CAD build for the part. Positions are in the model's coordinates, mm. Face numbers are marked on the shaded views. A direction names the side the tool comes from. Give positions to 0.01 mm unless a question says otherwise; leave off trailing zeros. Write each loop counter-clockwise with the first axis right and the second up, starting at its lowest first coordinate (ties: lowest second). Pieces come first, ordered by that corner, then holes. Notation, with made-up numbers: (-14.75, 30.25) -> (44.25, 30.25) arc R20 ccw to (44.25, 58.25) -> close; hole circle Ø5 at (72, -23). An arc over 180 degrees is marked (long way). Answer as a JSON object with one key per item and string values.
```python
from build123d import *

# Parameters (mm, degrees)
BOSS_EXTRUDE1_DEPTH                      = 38
BOSS_EXTRUDE3_DEPTH                      = 26
FILLET1_R                                = 6
CBORE_FOR_M30_HEX_HEAD_BOLT2_D           = 38
CBORE_FOR_M30_HEX_HEAD_BOLT2_CBORE_D     = 57
CBORE_FOR_M30_HEX_HEAD_BOLT2_CBORE_DEPTH = 1
SKETCH17_W                               = 26
SKETCH17_H                               = 18.384776311
CUT_EXTRUDE3_DEPTH                       = 180.605122421


with BuildPart() as part:
    # Sketch1 → Boss-Extrude1 (new body, symmetric)
    with BuildSketch(Plane.XY):
        Polygon((38, 139), (127, 50), (127, 0), (0, 0), (0, 139), align=None)
    extrude(amount=BOSS_EXTRUDE1_DEPTH, both=True)

    # Sketch3 → Boss-Extrude3 (add)
    with BuildSketch(Plane(origin=(0, 0, 0), x_dir=(1, 0, 0), z_dir=(0, 1, 0))):
        with BuildLine():
            Line((0, 38), (76, 38))
            Line((76, 38), (76, 89))
            ThreePointArc((76, 89), (38, 127), (0, 89))
            Line((0, 89), (0, 38))
        make_face()
        with BuildLine():
            Line((0, -38), (76, -38))
            Line((76, -38), (76, -89))
            ThreePointArc((76, -89), (38, -127), (0, -89))
            Line((0, -89), (0, -38))
        make_face()
    extrude(amount=BOSS_EXTRUDE3_DEPTH)

    # Fillet1
    fillet1_edges = [part.edges().sort_by_distance(p)[0] for p in [
        (76, 13, -38),
        (0, 26, -63.5),
        (38, 26, -38),
        (76, 26, -63.5),
        (38, 26, -127),
        (76, 13, 38),
        (0, 26, 63.5),
        (38, 26, 127),
        (76, 26, 63.5),
        (38, 26, 38),
        (0, 82.5, 38),
        (0, 82.5, -38),
    ]]
    fillet(fillet1_edges, radius=FILLET1_R)

    # CBORE for M30 Hex Head Bolt2 (through all)
    with Locations(Plane(origin=(0, 26, 0), x_dir=(1, 0, 0), z_dir=(0, 1, 0))):
        with Locations((38, -89), (38, 89)):
            CounterBoreHole(CBORE_FOR_M30_HEX_HEAD_BOLT2_D / 2, CBORE_FOR_M30_HEX_HEAD_BOLT2_CBORE_D / 2, CBORE_FOR_M30_HEX_HEAD_BOLT2_CBORE_DEPTH)

    # Sketch17 → Cut-Extrude3 (cut, through all)
    with BuildSketch(Plane(origin=(-63.5, 63.5, 0), x_dir=(0, 0, -1), z_dir=(-0.707106781, 0.707106781, 0))):
        with Locations((0, -115.965512115)):
            Rectangle(SKETCH17_W, SKETCH17_H)
    extrude(amount=-CUT_EXTRUDE3_DEPTH, mode=Mode.SUBTRACT)


solid = part.part
```
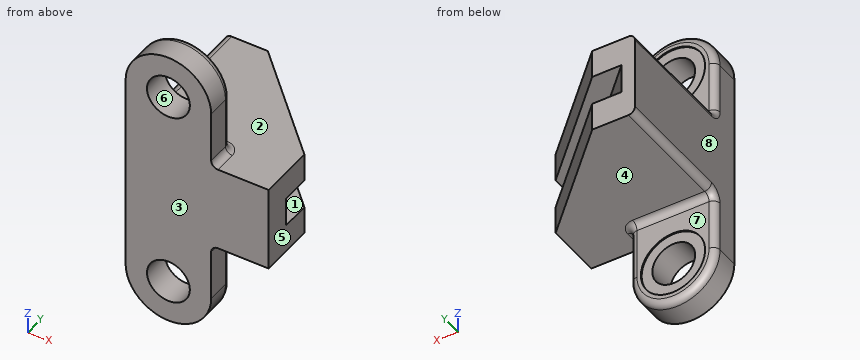
1) Slice it at C-C (x = 98.5). List the corners of the cut face in (y, z).
Model answer:
{"outline": "(0, -38) -> (78.5, -38) -> (78.5, -13) -> (52.5, -13) -> (52.5, 13) -> (78.5, 13) -> (78.5, 38) -> (0, 38) -> close"}
2) Slice it at B-B (y = 118). List the corners of the cut face in (x, z).
Model answer:
{"outline": "(0, -32) arc R6 ccw to (6, -38) -> (59, -38) -> (59, -13) -> (33, -13) -> (33, 13) -> (59, 13) -> (59, 38) -> (6, 38) arc R6 ccw to (0, 32) -> close"}
3) Pin check, flat tips, straight feed: pin 1 (1 mm diameter, centred on x = 108, z = -10, fed in from -Y); pin 2 (6 mm diameter, centred on y = 13, z = 64, fed in from +X); pin 3 (5 mm diameter, centred on x = 20, y = 84, fed in from +Z); pin 4 (19 mm diameter, centred on x = 38.5, z = -78.5, fed in from +Y). Stop position of each tip, or through.
Model answer:
{"pin 1": "stops at y = 0", "pin 2": "stops at x = 76", "pin 3": "stops at z = 38", "pin 4": "stops at y = 25"}
4) Slice it at D-D (z = -18.5). List the corners of the cut face in (x, y).
Model answer:
{"outline": "(0, 0) -> (127, 0) -> (127, 50) -> (38, 139) -> (0, 139) -> close"}
5) Wall check: probe 1 along Z at (x, y) = (38, 8.25); probe 2 along X at (y, z) = (14.5, -89); probe 3 along Z at (x, y) = (36, 7). Give the ranges that are in metal, low to high.
Model answer:
{"probe 1": "z = -127 to -108, -70 to 70, 108 to 127", "probe 2": "x = 0 to 19, 57 to 76", "probe 3": "z = -126.95 to -107.89, -70.11 to 70.11, 107.89 to 126.95"}
6) Slice it at A-A (y = 14.5). List the corners of the cut face in (x, z), then the cut area to 3 significant figures.
Model answer:
{"outline": "(0, -89) arc R38 ccw to (76, -89) -> (76, -44) arc R6 cw to (82, -38) -> (127, -38) -> (127, 38) -> (82, 38) arc R6 cw to (76, 44) -> (76, 89) arc R38 ccw to (0, 89) -> close; hole circle Ø38 at (38, -89); hole circle Ø38 at (38, 89)", "area": "19,700 mm2"}
7) 3-axis set-ups, long thin cutter, end or side, ignore diameter. For the marked faces 1, 2, 3, 4 and 5: which of +Z, -Z, +X, -X, +Y, -Y reach the whole face in a straight line?
Model answer:
{"face 1": "+X, +Y", "face 2": "+Z, +X, +Y", "face 3": "+Z, -Z, +X, -X, -Y", "face 4": "-Z, +X, +Y", "face 5": "+Z, -Z, +X, +Y, -Y"}
8) Mould opens along X. For the marked faces 6, 7 and 8 say: released by +X, released by -X, zero draft, split by the parting line, or undercut.
Model answer:
{"face 6": "undercut", "face 7": "zero draft", "face 8": "released by -X"}
